```python
from build123d import *

# Parameters (mm, degrees)
F2_R = 33.3375
F4_T = -2.86990282


with BuildPart() as f3:
    # F3: sweep along a path in F0
    with BuildLine(Plane.XZ) as f3_path:
        Line((-572.8366216311, 208.4954793713), (-84.1721266095, 30.6361486408))
        ThreePointArc((-84.1721266095, 30.6361486408), (1.3608319451, 7.7176614698), (89.5741061999, 0))
        Line((89.5741061999, 0), (644.3205312256, 0))
        ThreePointArc((644.3205312256, 0), (710.6278368734, 4.3460104221), (775.8006061377, 17.3096802452))
        Line((775.8006061377, 17.3096802452), (1128.2867717916, 111.7580636753))
    # F2 (on line) → F3 (sweep)
    with BuildSketch(Plane(origin=(-572.8366216311, 0, 208.4954793713), x_dir=(0, -1, 0), z_dir=(-0.9396926208, 0, 0.3420201433))):
        Circle(F2_R)
    sweep(path=f3_path.line)

    # F4
    f4_openings = [f3.faces().sort_by_distance(p)[0] for p in [
        (-572.836622, 0, 208.495479),
        (1128.286772, 0, 111.758064),
    ]]
    offset(amount=F4_T, openings=f4_openings)


solid = f3.part
```
Model file for the job. Use its own axes, mm. A direction names the side the tool comes from. Give positions to 0.01 mm unless a question says otherwise; leave off trailing zeros. Loops run counter-clockwise (first coordinate to the right, second up) from the corner with the lowest first, then second, coordinate; pieces in that order, holes last. Notation, with made-up numbers: (-9.75, -38) - (13.25, -38) arc R28 ccw to (13.25, -20) - close; hole circle Ø10 at (11.25, -6.5). An arc over 180 degrees is marked (long way). One line per item, written item: value. Start each with the question number.
1. Which spindle directions (+Z, -Z, +X, -X, +Y, -Y) get a long thin tool onto all of the face, cutting with end or side? Do faces 1 (the flat face through (-577.85, 27.01, 194.72)), 2 (the cylindrical face through (370.83, -31.8, -10.01)). Say none if no direction does.
2. Pull direction Y, two halves, no side cores. Call faces 3 (the cylindrical face through (370.83, -16.38, -25.69)), 4 (the cylindrical face through (-314.968, -15.383, 146.113)), 5 (the flat face through (1135.277, 14.661, 85.67)): pulls with the +Y half, pulls with the -Y half, needs draft (parallel to the pull), parting line crosses it, or undercut.
3. Probe L1, parallel to Z at x = 308, y = -4.5; L2, parallel to Z at x = 208, y = 0; L3, parallel to Y at x = 1014, z = 61.5. List the from-to ranges inside material, lowest first. Write a range as from..to.
4. Slice it at B-B (x = 193.5). List the corners of the cut face in (y, z) (1 decimal), plus the area to 3 significant figures.
5. Pin check, flat tips, straight feed: pin 1 (2 mm diameter, centred on x = 212, y = 0.5, fed in from -Z); pin 2 (8 mm diameter, centred on x = -293.5, z = 119, fed in from +Y); pin 3 (1.5 mm diameter, centred on x = 41, y = -10, fed in from +Z). Stop position of each tip, or through.
6. Slice it at A-A (y = 5.5). List the corners of the cut face in (x, z).
Solution:
1. face 1: +Z, -X, +Y, -Y
1. face 2: none
2. face 3: undercut
2. face 4: parting line crosses it
2. face 5: needs draft
3. L1: z = -33.03..-30.13, 30.13..33.03
3. L2: z = -33.34..-30.47, 30.47..33.34
3. L3: y = -27.42..-23.84, 23.84..27.42
4. outline: circle Ø66.7 at (0, 0); hole circle Ø60.9 at (0, 0)
4. area: 575 mm^2
5. pin 1: stops at z = -33.34
5. pin 2: stops at y = 32.5
5. pin 3: stops at z = 34.53
6. outline: (-584.08, 177.6) - (-95.42, -0.26) arc R540.88 ccw to (89.57, -32.88) - (644.32, -32.88) arc R540.88 ccw to (784.31, -14.45) - (1136.8, 80) - (1136.04, 82.81) - (783.56, -11.64) arc R537.97 cw to (644.32, -29.97) - (89.57, -29.97) arc R537.97 cw to (-94.42, 2.48) - (-583.09, 180.34) - close; (-562.59, 236.66) - (-73.92, 58.8) arc R478.03 ccw to (89.57, 29.97) - (644.32, 29.97) arc R478.03 ccw to (768.04, 46.26) - (1120.53, 140.7) - (1119.78, 143.52) - (767.29, 49.07) arc R475.12 cw to (644.32, 32.88) - (89.57, 32.88) arc R475.12 cw to (-72.93, 61.53) - (-561.59, 239.39) - close
